Input: part model. Units: mm. Frame: model coordinates. Face numbers are marked on the shaded views. A direction names the side the tool comes from. Round coordinates to 2 decimals unless told otherwise and drop trailing zeros. Loops run counter-clockwise (first coordinate to the right, second up) from the corner with the lowest first, then second, coordinate; pieces in that order, holes last. Notation, with made-up numbers: (-22.75, 12.5) -> (17.25, 12.5) arc R31 cw to (17.25, 43.5) -> close; hole circle Ø2 at (38.5, 20). An arc over 180 degrees is marked (long way). Answer as a JSON object with one key per item and string values.
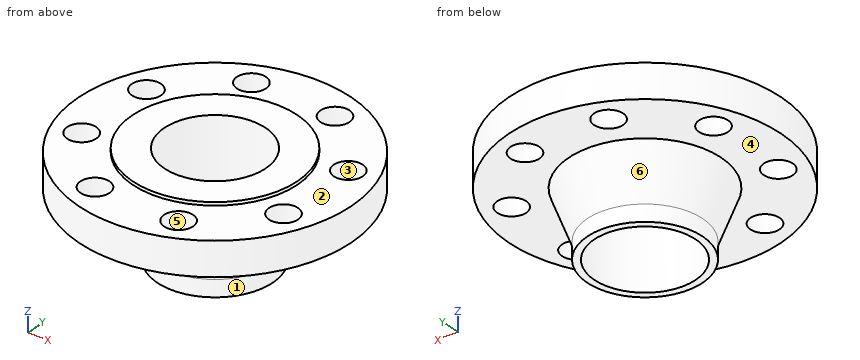
Autodesk Inventor part; units mm, degrees
ref_plane "YZ Plane" through (0, 0, 0) normal (1, 0, 0) x (0, 1, 0)
ref_plane "XZ Plane" through (0, 0, 0) normal (0, 1, 0) x (-1, 0, 0)
ref_plane "XY Plane" through (0, 0, 0) normal (0, 0, 1) x (1, 0, 0)
sketch "Sketch1" plane through (0, 0, 0) normal (0, 0, 1) x (1, 0, 0)
  circle A0 centre (0, 0) radius 104.775
  dimension "d_externo" = 209.55
extrude "Diametro externo" add sketch "Sketch1" against normal blind 28.448
sketch "Sketch2" plane through (0, 0, 0) normal (0, 0, 1) x (1, 0, 0)
  circle A0 centre (0, 0) radius 104.775
  circle A1 centre (0, 0) radius 63.5
  dimension "d_resaltado" = 127
extrude "Resaltado" cut sketch "Sketch2" against normal blind 2.5
sketch "Sketch3" plane through (0, 0, 0) normal (0, 1, 0) x (-1, 0, 0)
  line L0 (-104.775, -28.448) -> (104.775, -28.448) construction
  line L1 (63.5, 0) -> (-63.5, 0) construction
  line L2 (0, -83.82) -> (0, 13.97)
  line L3 (0, -28.448) -> (0, -79.248)
  line L4 (0, -79.248) -> (44.45, -79.248)
  line L5 (44.45, -79.248) -> (44.45, -66.548)
  line L6 (44.45, -66.548) -> (58.674, -28.448)
  line L7 (58.674, -28.448) -> (0, -28.448)
  point P0 (0, 0)
  point P1 (0, -28.448)
  point P2 (0, -79.248)
  dimension "dia_a" = 88.9
  dimension "dia_m" = 117.348
  dimension "d8" = 12.7
  dimension "altura_h" = 79.248
revolve "Cuello" add sketch "Sketch3" angle 360 about axis through (0, 0, -10) along (0, 0, 1)
sketch "Sketch4" plane through (0, 0, 0) normal (0, 0, 1) x (1, 0, 0)
  circle A0 centre (0, 0) radius 38.989
  dimension "d_interior" = 77.978
extrude "Diametro interior" cut sketch "Sketch4" against normal through all
sketch "Sketch5" plane through (0, 0, 0) normal (0, 0, 1) x (1, 0, 0)
  line L0 (0, -106.68) -> (0, 106.68) construction
  circle A0 centre (0, 0) radius 84.074 construction
  line L1 (0, 0) -> (32.1737, 77.6742) construction
  dimension "BCD" = 168.148
  dimension "ang_a1" = 22.5
hole "Agujero union" at (32.1737, 77.6742, 0) direction (0, 0, -1) diameter 22.352 end through all
pattern_circular "Patron agujero" count 8 over 360 about axis through (0, 0, -10) along (0, 0, 1) of "Agujero union"
sketch3d "Sketch6"
feature "RANURA_ORING:1" [suppressed]
equation "\"d8\" = -0.25 * espesor + 0.25 * altura_h"
properties part number "ej_iLogic" material "Steel"
1) Ray query, probe 1 along Y at (x, z) = (-85.5, -28) (3 decimals); probe 2 along X at (y, z) = (-30, -13); probe 3 along Y at (x, z) = (-78, -8.5). Return the intervals inside material, ascending.
Output:
{"probe 1": "y = -60.56 to -40.152, -24.195 to 24.195, 40.152 to 60.56", "probe 2": "x = -100.39 to -88.64, -66.71 to -24.9, 24.9 to 66.71, 88.64 to 100.39", "probe 3": "y = -69.96 to -43.34, -21 to 21, 43.34 to 69.96"}
2) Section D-D, the plane x = -77. Output: boundary loops of the cut face in (y, z).
Output:
{"outline": "(-71.05, -28.45) -> (-43.33, -28.45) -> (-43.33, -2.5) -> (-71.05, -2.5) -> close; (-21.02, -28.45) -> (21.02, -28.45) -> (21.02, -2.5) -> (-21.02, -2.5) -> close; (43.33, -28.45) -> (71.05, -28.45) -> (71.05, -2.5) -> (43.33, -2.5) -> close"}
3) Section C-C, the plane z = -24. Count the separate pieces of the cut face and the enclosed holes in it, plus the area to 3 significant figures.
Output:
{"separate pieces": "1", "enclosed holes": "9", "area": "26,600 mm^2"}
4) Reachability of the marked faces 1, 2 and 3 from +Z, -Z, +X, -X, +Y, -Y: full face, straight path, thin tool, end or side. Return the list, or none.
Output:
{"face 1": "-Z", "face 2": "+Z", "face 3": "+Z, -Z"}
5) Contact query for flat-ended pins moving along their axis: P1, Ø1, axis at y = 50.5, z = -16, coming from the -X side (3 decimals); P2, Ø2, axis at x = -36.5, z = -60.5, coming from the -Y side; P3, Ø13.5, axis at x = -77.67, y = 32.17, coming from the -Z side; P4, Ø5, axis at x = -59, y = -41, coming from the -Z side. Output: stop coordinate, or through.
Output:
{"P1": "stops at x = -92.075", "P2": "stops at y = -30.49", "P3": "passes through", "P4": "stops at z = -28.45"}
6) Section A-A, the plane y = 0. Output: boundary loops of the cut face in (x, z) (3 decimals).
Output:
{"outline": "(-104.775, -28.448) -> (-58.674, -28.448) -> (-44.45, -66.548) -> (-44.45, -79.248) -> (-38.989, -79.248) -> (-38.989, 0) -> (-63.5, 0) -> (-63.5, -2.5) -> (-104.775, -2.5) -> close; (38.989, -79.248) -> (44.45, -79.248) -> (44.45, -66.548) -> (58.674, -28.448) -> (104.775, -28.448) -> (104.775, -2.5) -> (63.5, -2.5) -> (63.5, 0) -> (38.989, 0) -> close"}
7) Draft query along Y for the marked faces 4, 5 and 6. Return one class per face: +Y half, -Y half, draft (parallel to the pull), parting line (faces both ways), or undercut.
Output:
{"face 4": "draft", "face 5": "undercut", "face 6": "parting line"}
